Solid Edge part; units mm, degrees
sketch "Sketch1" plane through (0, 0, 0) normal (0, 1, 0) x (-1, 0, 0)
  circle A0 centre (16.756, -24.8845) radius 2.25
  circle A1 centre (27.4161, 12.1803) radius 2.25
  circle A2 centre (-7.2345, 29.1146) radius 2.25
  circle A3 centre (-21.5968, -20.8226) radius 2.25
  circle A4 centre (0, -32) radius 2.8
  circle A5 centre (0, 32) radius 2.8
  circle A6 centre (0, 0) radius 39
  circle A7 centre (-32, 0) radius 2.8
  circle A8 centre (32, 0) radius 2.8
  circle A9 centre (-24.2565, 17.6529) radius 2.25
  circle A10 centre (13.1726, 26.9533) radius 2.25
  circle A11 centre (28.8313, -8.2921) radius 2.25
  circle A12 centre (0, 0) radius 17.5
extrude "Protrusion1" add sketch "Sketch1" along normal blind 15
sketch "Sketch2" plane through (0, 15, 0) normal (0, 1, 0) x (-1, 0, 0)
  circle A0 centre (27.4161, 12.1803) radius 2.25
  circle A1 centre (32, 0) radius 2.8
  circle A2 centre (13.1726, 26.9533) radius 2.25
  circle A3 centre (16.756, -24.8845) radius 2.25
  circle A4 centre (28.8313, -8.2921) radius 2.25
  circle A5 centre (0, -32) radius 2.8
  arc A6 (4.5655, 16.894) -> (-4.4574, -16.9228) centre (0, 0) cw
  line L0 (-4.4574, -16.9228) -> (-10, -37.6962)
  arc A7 (10.1123, 37.6662) -> (-10, -37.6962) centre (0, 0) cw
  line L1 (10.1123, 37.6662) -> (10, 37.262)
  line L2 (10, 37.262) -> (4.5655, 16.894)
extrude "ExtrudedCutout_1" cut sketch "Sketch2" along normal mid plane 476
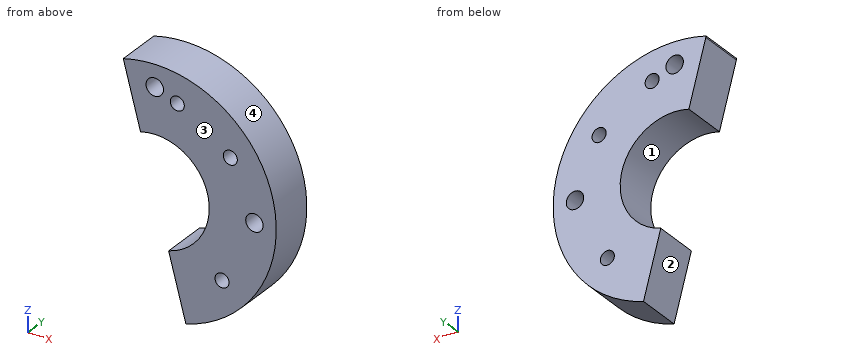
Input: part model. Units: mm. Frame: model coordinates. Face numbers are marked on the shaded views. Give positions to 0.01 mm unless a question says otherwise; leave off trailing zeros. Write each loop counter-clockwise with the first axis right and the second up, starting at its lowest first coordinate (ties: lowest second). Pieces come first, ordered by that corner, then holes. Notation, with made-up numbers: M 19,51.25 L 77,51.25 A21 cw 77,59.25 Z; hole C 48,64.25 d9. An arc over 180 degrees is marked long. Write item = value, one per line. Start each with the question number.
1) Cut plane B-B on x = 32. Return the cut outline in (y, z), then the cut area to 3 significant figures.
2) Cut plane D-D on z = -15.5. Return the cut outline in (x, y).
3) Draft query along Z for the marked faces 1, 2, 3 and 4. Return one class per face: +Z half, -Z half, draft (parallel to the pull), parting line (faces both ways), or undercut.
4) Material intervals for line 1 along X through (y, z) = (6.5, 34); line 2 along X through (y, z) = (4.75, -22); line 3 along Z through (x, y) = (32, 4), sorted ascending. Write a range as [from, to].
5) First-contact query: pin 1 Ø3.5 at (x, z) = (24.26, 17.65) entering from -Y; pin 2 Ø8 at (x, y) = (26.5, 8.5) entering from -Z; pin 3 Ø1.5 at (y, z) = (12, 28) entering from -X; pin 4 Ø5 at (x, y) = (14, 5.5) entering from -Z. Flat tips, straight axial feed; report the tip coordinate or a pass-through.
6) Cut plane A-A on z = 0. Return the cut outline in (x, y).
Solved:
q1.outline = M 0,-22.29 L 15,-22.29 L 15,-2.8 L 0,-2.8 Z; M 0,2.8 L 15,2.8 L 15,22.29 L 0,22.29 Z
q1.area = 585 mm2
q2.outline = M 8.12,0 L 35.79,0 L 35.79,15 L 8.12,15 Z
q3.face_1 = undercut
q3.face_2 = -Z half
q3.face_3 = draft
q3.face_4 = parting line
q4.line_1 = [-9.13, -1.96], [1.96, 19.1]
q4.line_2 = [5.81, 19.68], [23.51, 32.2]
q4.line_3 = [-22.29, -2.8], [2.8, 22.29]
q5.pin_1 = through
q5.pin_2 = -31.86
q5.pin_3 = -7.73
q5.pin_4 = -37.27
q6.outline = M 17.5,0 L 29.2,0 L 29.2,15 L 17.5,15 Z; M 34.8,0 L 39,0 L 39,15 L 34.8,15 Z
